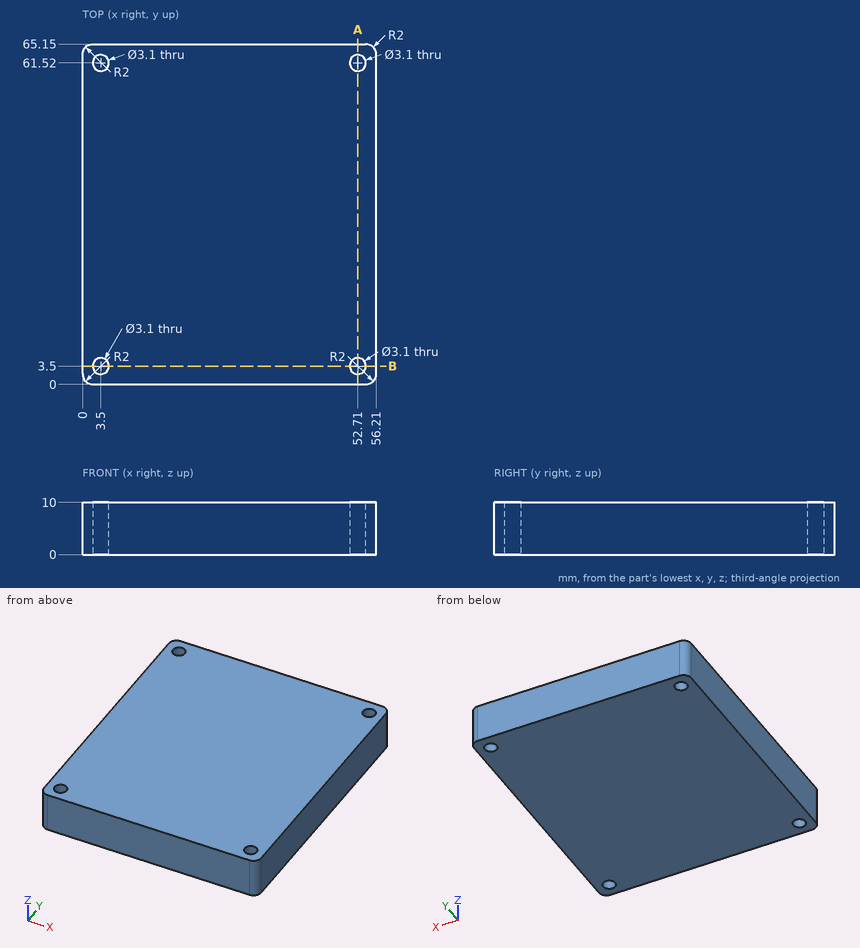
Check sheet for the drawn part. Datum: minimum x, y, z corner. Units: mm. Coordinates: 2 decimals unless noted, no trailing zeros. Write each loop counter-clockwise with the first axis right and the second up, starting at its lowest first coordinate (ties: lowest second). Pieces come first, ordered by that corner, then holes. Notation, with made-up numbers: M 1.25,84 L 8.25,84 A15 ccw 8.25,92 Z; hole C 51,74 d4. An arc over 180 degrees is marked long. Use a Markdown table: item, result.
Q1. Sectioned sample at B-B, the plane y = 3.5. Record the boundary of the cut face in (x, z).
Reply:
| item | result |
|---|---|
| outline | M 0,0 L 1.95,0 L 1.95,10 L 0,10 Z; M 5.05,0 L 51.16,0 L 51.16,10 L 5.05,10 Z; M 54.26,0 L 56.21,0 L 56.21,10 L 54.26,10 Z |
Q2. Go/stop test with a flat-tipped pin: P1, Ø2.5, axis at x = 52.71, y = 61.52, coming from the -Z side. Record where the tip stops, or that it passes through.
Reply:
| item | result |
|---|---|
| P1 | passes through |
Q3. Thickness scan on line 1 (Y direction, x = 52.71, z = 2); line 2 (X direction, y = 4, z = 7.5); line 3 (Y direction, x = 3, z = 2). Record the ranges inside material, lowest first.
Reply:
| item | result |
|---|---|
| line 1 | y = 0 to 1.95, 5.05 to 59.97, 63.07 to 65.15 |
| line 2 | x = 0 to 2.03, 4.97 to 51.24, 54.18 to 56.21 |
| line 3 | y = 0 to 2.03, 4.97 to 60.05, 62.99 to 65.15 |
Q4. Sectioned sample at A-A, the plane x = 52.71. Record the boundary of the cut face in (y, z).
Reply:
| item | result |
|---|---|
| outline | M 0,0 L 1.95,0 L 1.95,10 L 0,10 Z; M 5.05,0 L 59.97,0 L 59.97,10 L 5.05,10 Z; M 63.07,0 L 65.15,0 L 65.15,10 L 63.07,10 Z |
